Could you check a few things on this model? Use its own coordinates, in mm. Give positions to 0.01 mm unless a question says otherwise; leave off trailing zeros. Write each loop counter-clockwise with the first axis right and the second up, starting at its lowest first coordinate (ties: lowest second). Pieces come first, ordered by that corner, then holes. Notation, with made-up numbers: (62.25, 55) -> (76.25, 55) arc R16 ccw to (76.25, 82) -> close; hole circle Ø10 at (56.25, -33). An arc over 180 degrees is marked (long way). One line per question, with ' | ' between items.
from build123d import *

# Parameters (mm, degrees)
F0_W     = 482.6
F0_H     = 82.55
F1_DEPTH = 12.7
F2_R     = 3.175
F3_T     = -1.524
F4_R     = 3.175
F4_R_2   = 6.35
F4_W     = 17.4625
F4_H     = 41.275
F5_DEPTH = 12.7
F6_W     = 14.1732
F6_H     = 82.55
F7_DEPTH = 25.4


with BuildPart() as f1:
    # F0 (on Top) → F1 (new body)
    with BuildSketch(Plane.XY):
        Rectangle(F0_W, F0_H)
    extrude(amount=-F1_DEPTH)

    # F2
    f2_edges = [f1.edges().sort_by_distance(p)[0] for p in [
        (0, -41.275, 0),
    ]]
    fillet(f2_edges, radius=F2_R)

    # F3
    f3_openings = [f1.faces().sort_by_distance(p)[0] for p in [
        (0, 0, -12.7),
        (241.3, 0.08388, -6.361664),
        (0, 41.275, -6.35),
        (-241.3, 0.08388, -6.361664),
    ]]
    offset(amount=F3_T, openings=f3_openings)

    # F4 (on face) → F5 (join)
    with BuildSketch(Plane.XY):
        with Locations((-114.3, -12.7)):
            Circle(F4_R)
        with Locations((-63.5, -12.7)):
            Circle(F4_R)
        with Locations((-12.7, -12.7)):
            Circle(F4_R)
        with Locations((38.1, -12.7)):
            Circle(F4_R)
        with Locations((88.9, -12.7)):
            Circle(F4_R)
        with Locations((-165.1, -12.7)):
            Circle(F4_R)
        with Locations((133.35, 0)):
            Circle(F4_R_2)
        with Locations((133.35, -25.4)):
            Circle(F4_R_2)
        with Locations((165.1, -12.7)):
            Rectangle(F4_W, F4_H)
    extrude(amount=F5_DEPTH)

    # F6 (on face) → F7 (cut)
    with BuildSketch(Plane.XY):
        with Locations((-234.2134, 0)):
            Rectangle(F6_W, F6_H)
        with Locations((234.2134, 0)):
            Rectangle(F6_W, F6_H)
    extrude(amount=-F7_DEPTH, mode=Mode.SUBTRACT)


solid = f1.part
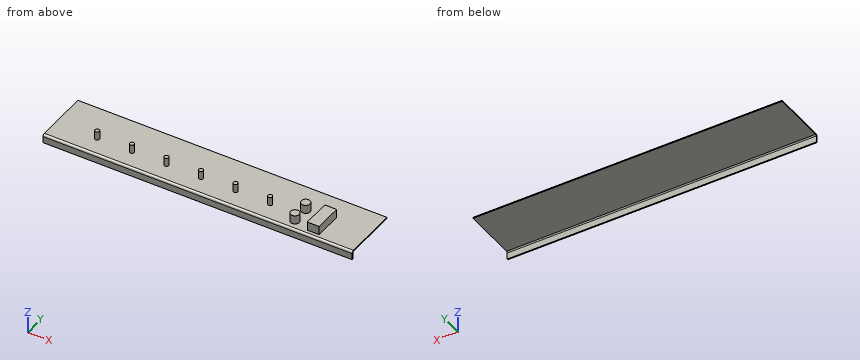
Q1. Imagine slicing it at B-B on x = -184. Please give me the cut outline in (y, z) (3 decimals).
Answer below:
outline: (-41.275, -12.7) -> (-39.751, -12.7) -> (-39.751, -3.175) arc R1.651 cw to (-38.1, -1.524) -> (41.275, -1.524) -> (41.275, 0) -> (-38.1, 0) arc R3.175 ccw to (-41.275, -3.175) -> close
Q2. Imagine slicing it at D-D on x = 133.35. Please give me the cut outline in (y, z) (3 decimals).
Answer below:
outline: (-41.275, -12.7) -> (-39.751, -12.7) -> (-39.751, -3.175) arc R1.651 cw to (-38.1, -1.524) -> (41.275, -1.524) -> (41.275, 0) -> (6.35, 0) -> (6.35, 12.7) -> (-6.35, 12.7) -> (-6.35, 0) -> (-19.05, 0) -> (-19.05, 12.7) -> (-31.75, 12.7) -> (-31.75, 0) -> (-38.1, 0) arc R3.175 ccw to (-41.275, -3.175) -> close
Q3. If I drill on line 1 along Z through (x, y) = (-28, -32.5); line 2 along X through (y, z) = (-27, 2.5); line 3 along Y through (x, z) = (-164, -10) (3 decimals), over which ranges is the centre line in solid material (lowest first)?
Answer below:
line 1: z = -1.52 to 0 | line 2: x = 127.2 to 139.5, 156.37 to 173.83 | line 3: y = -41.275 to -39.751
Q4. Imagine slicing it at C-C on y = -25.4. Please give me the cut outline in (x, z).
Answer below:
outline: (-227.13, -1.52) -> (227.13, -1.52) -> (227.13, 0) -> (173.83, 0) -> (173.83, 12.7) -> (156.37, 12.7) -> (156.37, 0) -> (139.7, 0) -> (139.7, 12.7) -> (127, 12.7) -> (127, 0) -> (-227.13, 0) -> close
Q5. Imagine slicing it at A-A on z = 7.5. Count the separate pieces of the cut face and the enclosed holes in it, and give its area (3 significant figures).
Answer below:
separate pieces: 9 | enclosed holes: 0 | area: 1,160 mm^2
Q6. Will these pins go through, and if not, where does the flat tip stop? pin 1 (5 mm diameter, centred on x = -14.5, z = -10, fed in from +Y); pin 2 (8 mm diameter, centred on x = 163, y = -22, fed in from -Z); pin 3 (6.5 mm diameter, centred on y = -4, z = 4.5, fed in from +X).
Answer below:
pin 1: stops at y = -39.75 | pin 2: stops at z = -1.52 | pin 3: stops at x = 173.83
